from build123d import *

# Parameters (mm, degrees)
SKETCH001_W             = 60
SKETCH001_H             = 15
PAD001_DEPTH            = 3
CHAMFER_SIZE            = 1
SKETCH005_R             = 1.6
POCKET002_DEPTH         = 3.001
BODY001_PLACEMENT_ANGLE = 90.00001


with BuildPart() as part:
    # Sketch001 → Pad001 (new body)
    with BuildSketch(Plane.YZ):
        with Locations((0, 2.5)):
            Rectangle(SKETCH001_W, SKETCH001_H)
    extrude(amount=-PAD001_DEPTH)

    # Chamfer
    chamfer_edges = [part.edges().sort_by_distance(p)[0] for p in [
        (-1.5, 30, 10),
        (-1.5, -30, 10),
        (-1.5, -30, -5),
        (-1.5, 30, -5),
    ]]
    chamfer(chamfer_edges, length=CHAMFER_SIZE)

    # Sketch005 → Pocket002 (cut, through all)
    with BuildSketch(Plane.YZ):
        with Locations((-24, 5)):
            Circle(SKETCH005_R)
        with Locations((24, 5)):
            Circle(SKETCH005_R)
    extrude(amount=-POCKET002_DEPTH, mode=Mode.SUBTRACT)


with BuildPart() as part_1:
    # Body001 placement: moved
    add(part.part.rotate(Axis((0, 0, 0), (0, 0, 1)), BODY001_PLACEMENT_ANGLE))


solid = part_1.part
Can you work these out from the model? Positions are in its coordinate system, mm. Coordinates: 2 decimals unless noted, no trailing zeros. Write each loop counter-clockwise with the first axis right and the second up, starting at its lowest first coordinate (ties: lowest second). Pieces come first, ordered by that corner, then holes. Notation, with made-up numbers: (13, 19) - (32, 19) arc R19 ccw to (32, 31) - close; hole circle Ø4 at (46, 27). An arc over 180 degrees is marked (long way). Return JSON: item names as keys, results as strings. Group by question number.
Item 1: If we section it at A-A (z = 5): Write out the boundary of the cut face in (x, y).
Item 2: I'm going to push a flat-ended pin straight in: pin 1 Ø3 at (x, z) = (-24, 5) entering from +Y. Where does the tip first touch, or does it pass through?
Item 3: We'd pull the mould along X, two halves only. Please class faces 1 (the face through (-30, -1, 2)), 2 (the face through (29.5, -1.5, -4.5)), 3 (the face through (-22.73, -1.48, 4.03)): pulls with the +X half, pulls with the -X half, needs draft (parallel to the pull), parting line crosses it, or undercut.
Item 4: If we section it at B-B (y = -1.05): Write out the boundary of the cut face in (x, z).
Item 5: Please list where these lines run through material, in increasing order: probe 1 along Z at (x, y) = (-24, -1.6); probe 2 along X at (y, z) = (-0.9, -4.5).
Return value:
{
 "1": {"outline": "(-30, -3) - (-25.6, -3) - (-25.6, 0) - (-30, 0) - close; (-22.4, -3) - (22.4, -3) - (22.4, 0) - (-22.4, 0) - close; (25.6, -3) - (30, -3) - (30, 0) - (25.6, 0) - close"},
 "2": {"pin 1": "passes through"},
 "3": {"face 1": "pulls with the -X half", "face 2": "pulls with the +X half", "face 3": "undercut"},
 "4": {"outline": "(-30, -4) - (-29, -5) - (29, -5) - (30, -4) - (30, 9) - (29, 10) - (-29, 10) - (-30, 9) - close; hole circle Ø3.2 at (-24, 5); hole circle Ø3.2 at (24, 5)"},
 "5": {"probe 1": "z = -5 to 3.4, 6.6 to 10", "probe 2": "x = -29.5 to 29.5"}
}
